Verification items for the finished model (mm, model axes). A direction names the side the tool comes from. Round coordinates to 2 decimals unless told otherwise and drop trailing zeros. Write each loop counter-clockwise with the first axis right and the second up, starting at its lowest first coordinate (ties: lowest second). Pieces come first, ordered by that corner, then holes. Notation, with made-up numbers: (-14.75, 62.25) - (37.25, 62.25) arc R14 ccw to (37.25, 73.25) - close; hole circle Ø11 at (-31, 39.25). An arc over 180 degrees is marked (long way). Answer as a JSON object with one key per item and string values.
```python
from build123d import *

# Parameters (mm, degrees)
ESBO_O1_W                = 170
ESBO_O1_H                = 96
RESSALTO_EXTRUS_O1_DEPTH = 6
CORTE_EXTRUS_O1_REACH    = 99.801
ESBO_O2_W                = 15.455454545
ESBO_O2_H                = 6
CORTE_EXTRUS_O2_REACH    = 99.801
ESBO_O3_W                = 6
ESBO_O3_H                = 13.714285714


with BuildPart() as part:
    # Esboço1 → Ressalto-extrusão1 (new body)
    with BuildSketch(Plane(origin=(0, 0, 0), x_dir=(0, 0, -1), z_dir=(1, 0, 0))):
        Rectangle(ESBO_O1_W, ESBO_O1_H)
    extrude(amount=RESSALTO_EXTRUS_O1_DEPTH)

    # Esboço2 → Corte-extrusão1 (cut, up to next)
    with BuildSketch(Plane(origin=(6, 0, 0), x_dir=(0, 0, -1), z_dir=(1, 0, 0)), mode=Mode.PRIVATE) as corte_extrus_o1_sk1:
        with Locations((0.002272727, 45)):
            Rectangle(ESBO_O2_W, ESBO_O2_H)
    corte_extrus_o1_tool1 = extrude(corte_extrus_o1_sk1.sketch, amount=-CORTE_EXTRUS_O1_REACH, mode=Mode.PRIVATE) & part.part
    # Esboço2 → Corte-extrusão1 (cut, up to next)
    with BuildSketch(Plane(origin=(6, 0, 0), x_dir=(0, 0, -1), z_dir=(1, 0, 0)), mode=Mode.PRIVATE) as corte_extrus_o1_sk2:
        with Locations((-30.907727273, 45)):
            Rectangle(ESBO_O2_W, ESBO_O2_H)
    corte_extrus_o1_tool2 = extrude(corte_extrus_o1_sk2.sketch, amount=-CORTE_EXTRUS_O1_REACH, mode=Mode.PRIVATE) & part.part
    # Esboço2 → Corte-extrusão1 (cut, up to next)
    with BuildSketch(Plane(origin=(6, 0, 0), x_dir=(0, 0, -1), z_dir=(1, 0, 0)), mode=Mode.PRIVATE) as corte_extrus_o1_sk3:
        with Locations((-61.817727273, 45)):
            Rectangle(ESBO_O2_W, ESBO_O2_H)
    corte_extrus_o1_tool3 = extrude(corte_extrus_o1_sk3.sketch, amount=-CORTE_EXTRUS_O1_REACH, mode=Mode.PRIVATE) & part.part
    # Esboço2 → Corte-extrusão1 (cut, up to next)
    with BuildSketch(Plane(origin=(6, 0, 0), x_dir=(0, 0, -1), z_dir=(1, 0, 0)), mode=Mode.PRIVATE) as corte_extrus_o1_sk4:
        with Locations((30.912272728, 45)):
            Rectangle(ESBO_O2_W, ESBO_O2_H)
    corte_extrus_o1_tool4 = extrude(corte_extrus_o1_sk4.sketch, amount=-CORTE_EXTRUS_O1_REACH, mode=Mode.PRIVATE) & part.part
    # Esboço2 → Corte-extrusão1 (cut, up to next)
    with BuildSketch(Plane(origin=(6, 0, 0), x_dir=(0, 0, -1), z_dir=(1, 0, 0)), mode=Mode.PRIVATE) as corte_extrus_o1_sk5:
        with Locations((61.822272728, 45)):
            Rectangle(ESBO_O2_W, ESBO_O2_H)
    corte_extrus_o1_tool5 = extrude(corte_extrus_o1_sk5.sketch, amount=-CORTE_EXTRUS_O1_REACH, mode=Mode.PRIVATE) & part.part
    # Esboço2 → Corte-extrusão1 (cut, up to next)
    with BuildSketch(Plane(origin=(6, 0, 0), x_dir=(0, 0, -1), z_dir=(1, 0, 0)), mode=Mode.PRIVATE) as corte_extrus_o1_sk6:
        with Locations((-61.817727273, -48)):
            Rectangle(ESBO_O2_W, ESBO_O2_H)
    corte_extrus_o1_tool6 = extrude(corte_extrus_o1_sk6.sketch, amount=-CORTE_EXTRUS_O1_REACH, mode=Mode.PRIVATE) & part.part
    # Esboço2 → Corte-extrusão1 (cut, up to next)
    with BuildSketch(Plane(origin=(6, 0, 0), x_dir=(0, 0, -1), z_dir=(1, 0, 0)), mode=Mode.PRIVATE) as corte_extrus_o1_sk7:
        with Locations((-30.907727273, -48)):
            Rectangle(ESBO_O2_W, ESBO_O2_H)
    corte_extrus_o1_tool7 = extrude(corte_extrus_o1_sk7.sketch, amount=-CORTE_EXTRUS_O1_REACH, mode=Mode.PRIVATE) & part.part
    # Esboço2 → Corte-extrusão1 (cut, up to next)
    with BuildSketch(Plane(origin=(6, 0, 0), x_dir=(0, 0, -1), z_dir=(1, 0, 0)), mode=Mode.PRIVATE) as corte_extrus_o1_sk8:
        with Locations((0.002272727, -48)):
            Rectangle(ESBO_O2_W, ESBO_O2_H)
    corte_extrus_o1_tool8 = extrude(corte_extrus_o1_sk8.sketch, amount=-CORTE_EXTRUS_O1_REACH, mode=Mode.PRIVATE) & part.part
    # Esboço2 → Corte-extrusão1 (cut, up to next)
    with BuildSketch(Plane(origin=(6, 0, 0), x_dir=(0, 0, -1), z_dir=(1, 0, 0)), mode=Mode.PRIVATE) as corte_extrus_o1_sk9:
        with Locations((30.912272728, -48)):
            Rectangle(ESBO_O2_W, ESBO_O2_H)
    corte_extrus_o1_tool9 = extrude(corte_extrus_o1_sk9.sketch, amount=-CORTE_EXTRUS_O1_REACH, mode=Mode.PRIVATE) & part.part
    # Esboço2 → Corte-extrusão1 (cut, up to next)
    with BuildSketch(Plane(origin=(6, 0, 0), x_dir=(0, 0, -1), z_dir=(1, 0, 0)), mode=Mode.PRIVATE) as corte_extrus_o1_sk10:
        with Locations((61.822272728, -48)):
            Rectangle(ESBO_O2_W, ESBO_O2_H)
    corte_extrus_o1_tool10 = extrude(corte_extrus_o1_sk10.sketch, amount=-CORTE_EXTRUS_O1_REACH, mode=Mode.PRIVATE) & part.part
    add(corte_extrus_o1_tool1.solids().sort_by_distance((6, 45, -0.002273))[0], mode=Mode.SUBTRACT)
    add(corte_extrus_o1_tool2.solids().sort_by_distance((6, 45, 30.907727))[0], mode=Mode.SUBTRACT)
    add(corte_extrus_o1_tool3.solids().sort_by_distance((6, 45, 61.817727))[0], mode=Mode.SUBTRACT)
    add(corte_extrus_o1_tool4.solids().sort_by_distance((6, 45, -30.912273))[0], mode=Mode.SUBTRACT)
    add(corte_extrus_o1_tool5.solids().sort_by_distance((6, 45, -61.822273))[0], mode=Mode.SUBTRACT)
    add(corte_extrus_o1_tool6.solids().sort_by_distance((6, -48, 61.817727))[0], mode=Mode.SUBTRACT)
    add(corte_extrus_o1_tool7.solids().sort_by_distance((6, -48, 30.907727))[0], mode=Mode.SUBTRACT)
    add(corte_extrus_o1_tool8.solids().sort_by_distance((6, -48, -0.002273))[0], mode=Mode.SUBTRACT)
    add(corte_extrus_o1_tool9.solids().sort_by_distance((6, -48, -30.912273))[0], mode=Mode.SUBTRACT)
    add(corte_extrus_o1_tool10.solids().sort_by_distance((6, -48, -61.822273))[0], mode=Mode.SUBTRACT)

    # Esboço3 → Corte-extrusão2 (cut, up to next)
    with BuildSketch(Plane(origin=(6, 0, 0), x_dir=(0, 0, -1), z_dir=(1, 0, 0)), mode=Mode.PRIVATE) as corte_extrus_o2_sk1:
        with Locations((82, -41.142857143)):
            Rectangle(ESBO_O3_W, ESBO_O3_H)
    corte_extrus_o2_tool1 = extrude(corte_extrus_o2_sk1.sketch, amount=-CORTE_EXTRUS_O2_REACH, mode=Mode.PRIVATE) & part.part
    # Esboço3 → Corte-extrusão2 (cut, up to next)
    with BuildSketch(Plane(origin=(6, 0, 0), x_dir=(0, 0, -1), z_dir=(1, 0, 0)), mode=Mode.PRIVATE) as corte_extrus_o2_sk2:
        with Locations((-82, -41.142857143)):
            Rectangle(ESBO_O3_W, ESBO_O3_H)
    corte_extrus_o2_tool2 = extrude(corte_extrus_o2_sk2.sketch, amount=-CORTE_EXTRUS_O2_REACH, mode=Mode.PRIVATE) & part.part
    # Esboço3 → Corte-extrusão2 (cut, up to next)
    with BuildSketch(Plane(origin=(6, 0, 0), x_dir=(0, 0, -1), z_dir=(1, 0, 0)), mode=Mode.PRIVATE) as corte_extrus_o2_sk3:
        with Locations((82, -13.712857143)):
            Rectangle(ESBO_O3_W, ESBO_O3_H)
    corte_extrus_o2_tool3 = extrude(corte_extrus_o2_sk3.sketch, amount=-CORTE_EXTRUS_O2_REACH, mode=Mode.PRIVATE) & part.part
    # Esboço3 → Corte-extrusão2 (cut, up to next)
    with BuildSketch(Plane(origin=(6, 0, 0), x_dir=(0, 0, -1), z_dir=(1, 0, 0)), mode=Mode.PRIVATE) as corte_extrus_o2_sk4:
        with Locations((82, 13.717142857)):
            Rectangle(ESBO_O3_W, ESBO_O3_H)
    corte_extrus_o2_tool4 = extrude(corte_extrus_o2_sk4.sketch, amount=-CORTE_EXTRUS_O2_REACH, mode=Mode.PRIVATE) & part.part
    # Esboço3 → Corte-extrusão2 (cut, up to next)
    with BuildSketch(Plane(origin=(6, 0, 0), x_dir=(0, 0, -1), z_dir=(1, 0, 0)), mode=Mode.PRIVATE) as corte_extrus_o2_sk5:
        with Locations((82, 41.147142857)):
            Rectangle(ESBO_O3_W, ESBO_O3_H)
    corte_extrus_o2_tool5 = extrude(corte_extrus_o2_sk5.sketch, amount=-CORTE_EXTRUS_O2_REACH, mode=Mode.PRIVATE) & part.part
    # Esboço3 → Corte-extrusão2 (cut, up to next)
    with BuildSketch(Plane(origin=(6, 0, 0), x_dir=(0, 0, -1), z_dir=(1, 0, 0)), mode=Mode.PRIVATE) as corte_extrus_o2_sk6:
        with Locations((-82, -13.712857143)):
            Rectangle(ESBO_O3_W, ESBO_O3_H)
    corte_extrus_o2_tool6 = extrude(corte_extrus_o2_sk6.sketch, amount=-CORTE_EXTRUS_O2_REACH, mode=Mode.PRIVATE) & part.part
    # Esboço3 → Corte-extrusão2 (cut, up to next)
    with BuildSketch(Plane(origin=(6, 0, 0), x_dir=(0, 0, -1), z_dir=(1, 0, 0)), mode=Mode.PRIVATE) as corte_extrus_o2_sk7:
        with Locations((-82, 13.717142857)):
            Rectangle(ESBO_O3_W, ESBO_O3_H)
    corte_extrus_o2_tool7 = extrude(corte_extrus_o2_sk7.sketch, amount=-CORTE_EXTRUS_O2_REACH, mode=Mode.PRIVATE) & part.part
    # Esboço3 → Corte-extrusão2 (cut, up to next)
    with BuildSketch(Plane(origin=(6, 0, 0), x_dir=(0, 0, -1), z_dir=(1, 0, 0)), mode=Mode.PRIVATE) as corte_extrus_o2_sk8:
        with Locations((-82, 41.147142857)):
            Rectangle(ESBO_O3_W, ESBO_O3_H)
    corte_extrus_o2_tool8 = extrude(corte_extrus_o2_sk8.sketch, amount=-CORTE_EXTRUS_O2_REACH, mode=Mode.PRIVATE) & part.part
    add(corte_extrus_o2_tool1.solids().sort_by_distance((6, -41.142857, -82))[0], mode=Mode.SUBTRACT)
    add(corte_extrus_o2_tool2.solids().sort_by_distance((6, -41.142857, 82))[0], mode=Mode.SUBTRACT)
    add(corte_extrus_o2_tool3.solids().sort_by_distance((6, -13.712857, -82))[0], mode=Mode.SUBTRACT)
    add(corte_extrus_o2_tool4.solids().sort_by_distance((6, 13.717143, -82))[0], mode=Mode.SUBTRACT)
    add(corte_extrus_o2_tool5.solids().sort_by_distance((6, 41.147143, -82))[0], mode=Mode.SUBTRACT)
    add(corte_extrus_o2_tool6.solids().sort_by_distance((6, -13.712857, 82))[0], mode=Mode.SUBTRACT)
    add(corte_extrus_o2_tool7.solids().sort_by_distance((6, 13.717143, 82))[0], mode=Mode.SUBTRACT)
    add(corte_extrus_o2_tool8.solids().sort_by_distance((6, 41.147143, 82))[0], mode=Mode.SUBTRACT)


solid = part.part
```
1. Material ranges on probe 1 along Z at (x, y) = (4.95, -15.5); probe 2 along Y at (x, z) = (1.8, -64), recorded low to high. Write a range as from..to.
Completed:
{"probe 1": "z = -79..79", "probe 2": "y = -45..42"}
2. Go/stop test with flat-tipped pins: pin 1 (1.8 mm diameter, centred on x = 4.5, y = 38.5, fed in from -Z); pin 2 (1.8 mm diameter, centred on x = 4.5, z = 58.5, fed in from +Y); pin 3 (1 mm diameter, centred on y = 16.5, z = 4.5, fed in from -X); pin 4 (1.8 mm diameter, centred on x = 4.5, z = -82, fed in from +Y). Record where each tip stops, or that it passes through.
Completed:
{"pin 1": "stops at z = -79", "pin 2": "stops at y = 42", "pin 3": "stops at x = 0", "pin 4": "stops at y = 34.29"}
3. Cross-section at A-A (z = -6). Record the boundary of the cut face in (x, y).
Completed:
{"outline": "(0, -45) - (6, -45) - (6, 42) - (0, 42) - close"}
4. Cross-section at B-B (y = 38.5). Record the boundary of the cut face in (x, z), plus the area to 3 significant figures.
Completed:
{"outline": "(0, -79) - (6, -79) - (6, 79) - (0, 79) - close", "area": "948 mm^2"}
5. Access from +Z, -Z, +X, -X, +Y, -Y to the whole of each face (thin tool, end or side, straight path). Record for faces 4 (the face through (3, -47, -7.73)), 5 (the face through (3, 45, 7.725)), 6 (the face through (3, 14, 79)).
Completed:
{"face 4": "+X, -X, -Y", "face 5": "+X, -X, +Y", "face 6": "+Z, +X, -X"}
6. Mould release check, pull along Z, two halves, no side actions. Record for faces 1 (the face through (3, 27, 85)), 2 (the face through (3, 45, -54.095)), 3 (the face through (6, 1, 1)): released by +Z, released by -Z, zero draft, split by the parting line, or undercut.
Completed:
{"face 1": "released by +Z", "face 2": "undercut", "face 3": "zero draft"}
